Source: CAD feature listing. Evaluate the final solid. Frame: model axes, mm. Face numbers are marked on the shaded views. A direction names the side the tool comes from. Round coordinates to 2 decimals unless told otherwise and drop trailing zeros. Order: outer loops, then holes, each group sorted by start corner. A loop starts at its lowest first (then second) coordinate and runs counter-clockwise, first axis right, second up. Notation, with made-up numbers: M 38,-9 L 77,-9 A25 cw 77,27 Z; hole C 36,-2 d4. An arc over 180 degrees is marked long. Answer as CSV lines item,"result". Start each with the question number.
Item 1: Section query A-A on y = 0. Return the cut outline in (x, z).
Item 2: Section query D-D on z = -15.25. Return the cut outline in (x, y), plus the area to 3 significant figures.
Item 3: Line query: line 1 (Y direction, x = -17.5, z = -0.4); line 2 (Z direction, x = -1, y = 3); line 3 (X direction, y = -3.5, z = -2.5). Output: solid intervals per line, ascending. Write a range as [from, to].
Item 4: First-contact query: P1, Ø0.7, axis at x = 15.5, z = -0.5, coming from the +Y side; P2, Ø1.5, axis at x = 12, y = 2.5, coming from the +Z side; P3, Ø5.5, axis at y = 15.5, z = -7, coming from the +X side; P4, Ø6, axis at x = -11.5, y = 14, coming from the +Z side. Flat tips, straight axial feed; report the tip coordinate or a pass-through.
Item 5: Set-up query: the marked faces 1, 2 and 3. Return all of +Z, -Z, +X, -X, +Y, -Y with unobstructed straight access to the full face (end or side cutting, diameter ignored); none if empty.
Item 6: Section query B-B on z = -3. Return the cut outline in (x, y), plus the area to 3 significant figures.
Item 7: Section query C-C on y = 9.5. Return the cut outline in (x, z), plus the area to 3 significant figures.
from build123d import *

# Parameters (mm, degrees)
F0_R      = 14
F5_DEPTH  = 19
F2_W      = 14.6
F2_H      = 5.053871
F6_DEPTH  = 16.51
F7_DEPTH  = 12.7
F3_R      = 2.1
F8_DEPTH  = 0.8636
F9_DEPTH  = 10
F10_DEPTH = 4
F4_R      = 4.5
F11_DEPTH = 1.5


with BuildPart() as f5:
    # F0 (on Top) → F5 (new body)
    with BuildSketch(Plane.XY):
        Circle(F0_R)
    extrude(amount=-F5_DEPTH)

    # F2 (on Top) → F6 (join)
    with BuildSketch(Plane.XY):
        with Locations((0, 14.473064)):
            Rectangle(F2_W, F2_H)
    extrude(amount=-F6_DEPTH)

    # F1 (on Top) → F7 (join)
    with BuildSketch(Plane.XY):
        with BuildLine():
            ThreePointArc((-8.6868, 10.979048), (0, 14), (8.6868, 10.979048))
            Line((8.6868, 10.979048), (8.6868, 12.55836))
            ThreePointArc((8.6868, 12.55836), (0, 15.27), (-8.6868, 12.55836))
            Line((-8.6868, 12.55836), (-8.6868, 10.979048))
        make_face()
    extrude(amount=-F7_DEPTH)

    # F3 (on Top) → F8 (join)
    with BuildSketch(Plane.XY):
        with BuildLine():
            Line((17.5, 3.5), (-17.5, 3.5))
            ThreePointArc((-17.5, 3.5), (-21, 0), (-17.5, -3.5))
            Line((-17.5, -3.5), (17.5, -3.5))
            ThreePointArc((17.5, -3.5), (21, 0), (17.5, 3.5))
        make_face()
        with Locations((-17.5, 0)):
            Circle(F3_R, mode=Mode.SUBTRACT)
        with Locations((17.5, 0)):
            Circle(F3_R, mode=Mode.SUBTRACT)
    extrude(amount=-F8_DEPTH)

    # F4 (on Top) → F9 (join)
    with BuildSketch(Plane.XY):
        Polygon((0.353553, -5.525126), (-2.474874, -8.353553), (-0.353553, -10.474874), (2.474874, -7.646447), align=None)
        with BuildLine():
            Line((-0.353553, -10.474874), (-2.474874, -8.353553))
            ThreePointArc((-2.474874, -8.353553), (-1.767767, -9.767767), (-0.353553, -10.474874))
        make_face()
        with BuildLine():
            ThreePointArc((2.474874, -7.646447), (1.767767, -6.232233), (0.353553, -5.525126))
            Line((0.353553, -5.525126), (2.474874, -7.646447))
        make_face()
    extrude(amount=F9_DEPTH)

    # F4 (on Top) → F10 (join)
    with BuildSketch(Plane.XY):
        with BuildLine():
            Line((2.474874, -7.646447), (-0.353553, -10.474874))
            ThreePointArc((-0.353553, -10.474874), (1.767767, -9.767767), (2.474874, -7.646447))
        make_face()
        with BuildLine():
            ThreePointArc((0.353553, -5.525126), (-1.767767, -6.232233), (-2.474874, -8.353553))
            Line((-2.474874, -8.353553), (0.353553, -5.525126))
        make_face()
    extrude(amount=F10_DEPTH)

    # F4 (on Top) → F11 (join)
    with BuildSketch(Plane.XY):
        with Locations((0, -8)):
            Circle(F4_R)
        with BuildLine():
            ThreePointArc((-0.353553, -10.474874), (-1.767767, -9.767767), (-2.474874, -8.353553))
            ThreePointArc((-2.474874, -8.353553), (-1.767767, -6.232233), (0.353553, -5.525126))
            ThreePointArc((0.353553, -5.525126), (1.767767, -6.232233), (2.474874, -7.646447))
            ThreePointArc((2.474874, -7.646447), (1.767767, -9.767767), (-0.353553, -10.474874))
        make_face(mode=Mode.SUBTRACT)
        with BuildLine():
            Line((2.474874, -7.646447), (-0.353553, -10.474874))
            ThreePointArc((-0.353553, -10.474874), (1.767767, -9.767767), (2.474874, -7.646447))
        make_face()
    extrude(amount=F11_DEPTH)


solid = f5.part
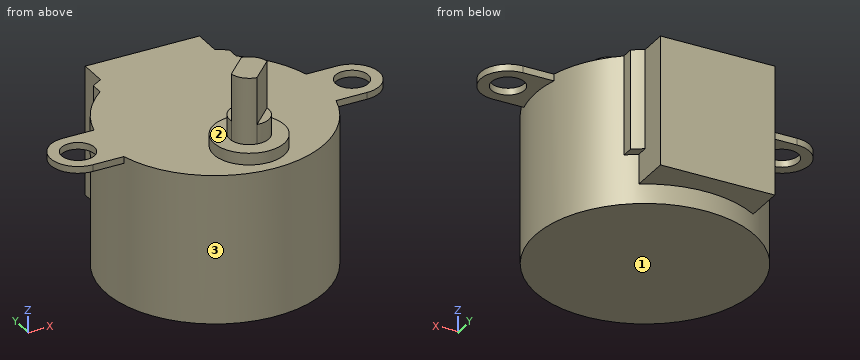
Results:
1,outline,"M -21,-0.86 L -19.6,-0.86 L -19.6,0 L -21,0 Z; M -15.4,-0.86 L -14,-0.86 L -14,-19 L 14,-19 L 14,-0.86 L 15.4,-0.86 L 15.4,0 L -15.4,0 Z; M 19.6,-0.86 L 21,-0.86 L 21,0 L 19.6,0 Z"
2,outline,"M -7.3,11.95 A14 ccw long 7.3,11.95 L 7.3,17 L -7.3,17 Z"
2,area,"669 mm^2"
3,line 1,"[-3.5, -2.1], [2.1, 3.5]"
3,line 2,"[-19, 0]"
3,line 3,"[-13.56, 13.56]"
4,P1,"y = 3.5"
4,P2,"z = 0"
4,P3,"x = 8.4"
4,P4,"through"
5,face 1,"-Z, +X, -X, +Y, -Y"
5,face 2,"+Z"
5,face 3,"-Z"
6,outline,"M -8.69,10.98 A14 ccw long 8.69,10.98 L 8.69,12.56 A15.27 ccw 7.3,13.41 L 7.3,17 L -7.3,17 L -7.3,13.41 A15.27 ccw -8.69,12.56 Z"
6,area,"673 mm^2"
7,outline,"M -10.28,-19 L 10.28,-19 L 10.28,0 L -10.28,0 Z"
7,area,"391 mm^2"
